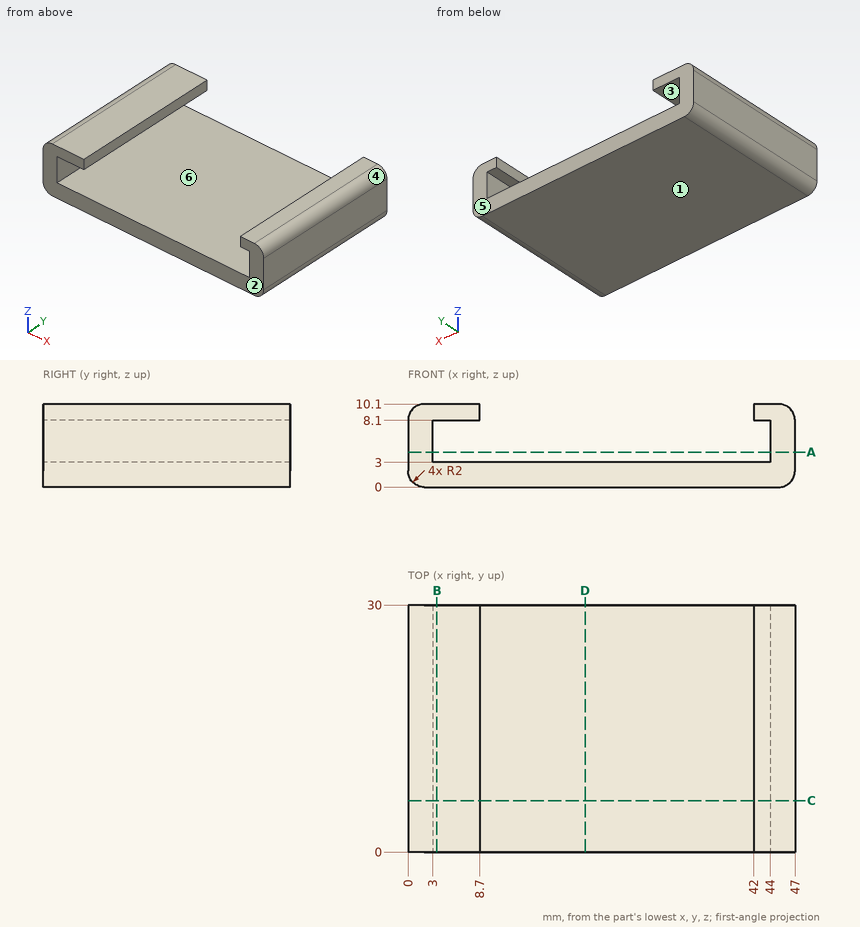
Source: three-view drawing plus pictorial views. Frame: mm from the lowest corner of the part. A direction names the side the tool comes from. Give positions to 0.01 mm unless a question says otherwise; leave off trailing zeros. Write each loop counter-clockwise with the first axis right and the second up, starting at its lowest first coordinate (ties: lowest second). Pieces come first, ordered by that corner, then holes. Notation, with made-up numbers: (79.25, -8.5) - (101.25, -8.5) arc R18 ccw to (101.25, 16.5) - close; hole circle Ø9 at (22, 3.25). An arc over 180 degrees is marked (long way). Write item = value, one per line. Start each with the question number.
1. Mould query, pull axis Z, two halves, no side actions, for the marked faces 1, 2, 3 and 4. Classes: released by +Z, released by -Z, zero draft, split by the parting line, or undercut.
2. Section query A-A, the plane z = 4.25. Output: boundary loops of the cut face in (x, y).
3. Section query B-B, the plane x = 3.5. Output: boundary loops of the cut face in (y, z).
4. Access query for the marked faces 5 and 6. Directions: +Z, -Z, +X, -X, +Y, -Y. A direction counts if a zero-diameter tool reaches every point of the face in a straight line with its end or side. Return the directions, or none.
5. First-contact query: pin 1 Ø6 at (x, y) = (31.5, 8) entering from +Z; pin 2 Ø3 at (x, y) = (18, 24.5) entering from -Z; pin 3 Ø1 at (y, z) = (10.5, 9) entering from -X; pin 4 Ø1.6 at (y, z) = (14, 9) entering from +X. Flat tips, straight axial feed; report the tip coordinate or a pass-through.
6. Section query C-C, the plane y = 6.25. Output: boundary loops of the cut face in (x, z).
7. Ray query, L1, parallel to X at y = 8.5, z = 7.5; L2, parallel to Z at x = 3.5, y = 2; L3, parallel to Z at x = 23, y = 11.75. Return the intervals inside material, ascending.
8. Section query D-D, the plane x = 21.5. Output: boundary loops of the cut face in (y, z), then the cut area to 3 significant figures.
Check sheet entries:
q1.face_1 = released by -Z
q1.face_2 = zero draft
q1.face_3 = undercut
q1.face_4 = released by +Z
q2.outline = (0, 0) - (3, 0) - (3, 30) - (0, 30) - close; (44, 0) - (47, 0) - (47, 30) - (44, 30) - close
q3.outline = (0, 0) - (30, 0) - (30, 3) - (0, 3) - close; (0, 8.1) - (30, 8.1) - (30, 10.1) - (0, 10.1) - close
q4.face_5 = +Z, -Z, +X, -X, +Y
q4.face_6 = +Y, -Y
q5.pin_1 = 3
q5.pin_2 = 0
q5.pin_3 = 0.04
q5.pin_4 = 47
q6.outline = (0, 2) arc R2 ccw to (2, 0) - (45, 0) arc R2 ccw to (47, 2) - (47, 8.1) arc R2 ccw to (45, 10.1) - (42, 10.1) - (42, 8.1) - (44, 8.1) - (44, 3) - (3, 3) - (3, 8.1) - (8.7, 8.1) - (8.7, 10.1) - (2, 10.1) arc R2 ccw to (0, 8.1) - close
q7.L1 = 0 to 3, 44 to 47
q7.L2 = 0 to 3, 8.1 to 10.1
q7.L3 = 0 to 3
q8.outline = (0, 0) - (30, 0) - (30, 3) - (0, 3) - close
q8.area = 90.0 mm2
